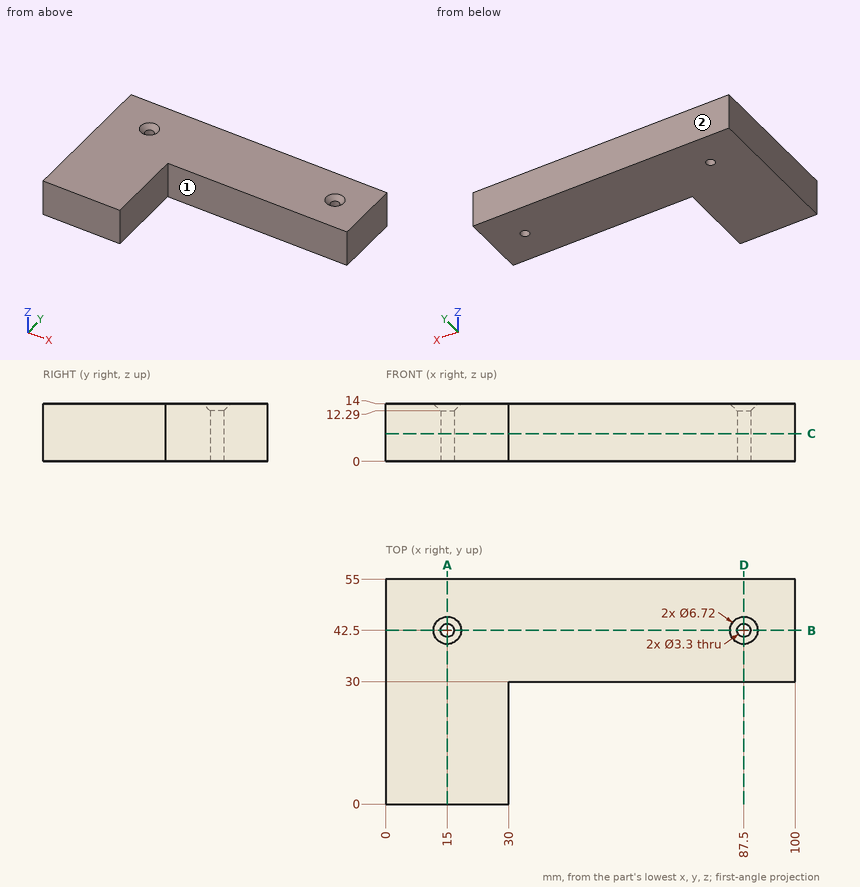
Could you check a few things on this drawing? It's one solid part, dimensions in mm from its lowest x, y, z. A direction names the side the tool comes from. Give positions to 0.01 mm unless a question says otherwise; leave off trailing zeros. Write each loop counter-clockwise with the first axis right and the second up, starting at its lowest first coordinate (ties: lowest second). Pieces come first, ordered by that corner, then holes. Notation, with made-up numbers: (35.5, 24.5) -> (87.5, 24.5) arc R16 cw to (87.5, 48.5) -> close; hole circle Ø5 at (-2.5, 63). An arc over 180 degrees is marked (long way). Answer as a JSON object with one key per item and string values.
Q1. Suppose I cut it at A-A on x = 15. Write out the boundary of the cut face in (y, z).
Taken from the geometry:
{"outline": "(0, 0) -> (40.85, 0) -> (40.85, 12.29) -> (39.14, 14) -> (0, 14) -> close; (44.15, 0) -> (55, 0) -> (55, 14) -> (45.86, 14) -> (44.15, 12.29) -> close"}
Q2. Suppose I cut it at B-B on y = 42.5. Write out the boundary of the cut face in (x, z).
Taken from the geometry:
{"outline": "(0, 0) -> (13.35, 0) -> (13.35, 12.29) -> (11.64, 14) -> (0, 14) -> close; (16.65, 0) -> (85.85, 0) -> (85.85, 12.29) -> (84.14, 14) -> (18.36, 14) -> (16.65, 12.29) -> close; (89.15, 0) -> (100, 0) -> (100, 14) -> (90.86, 14) -> (89.15, 12.29) -> close"}
Q3. Suppose I cut it at C-C on z = 6.75. Write out the boundary of the cut face in (x, y).
Taken from the geometry:
{"outline": "(0, 0) -> (30, 0) -> (30, 30) -> (100, 30) -> (100, 55) -> (0, 55) -> close; hole circle Ø3.3 at (15, 42.5); hole circle Ø3.3 at (87.5, 42.5)"}
Q4. Which directions (+Z, -Z, +X, -X, +Y, -Y) give clear straight access to the entire face, cutting with the end or side of a thin tool? Please do the marked faces 1 and 2.
Taken from the geometry:
{"face 1": "+Z, -Z, +X, -Y", "face 2": "+Z, -Z, +X, -X, +Y"}
Q5. Please list where these lines run through material, in increasing order: L1, parallel to X at y = 42.5, z = 2.5; L2, parallel to Y at x = 15, z = 4.25; L3, parallel to Y at x = 79, z = 6.25.
Taken from the geometry:
{"L1": "x = 0 to 13.35, 16.65 to 85.85, 89.15 to 100", "L2": "y = 0 to 40.85, 44.15 to 55", "L3": "y = 30 to 55"}
Q6. Suppose I cut it at D-D on x = 87.5. Write out the boundary of the cut face in (y, z), then the cut area to 3 significant figures.
Taken from the geometry:
{"outline": "(30, 0) -> (40.85, 0) -> (40.85, 12.29) -> (39.14, 14) -> (30, 14) -> close; (44.15, 0) -> (55, 0) -> (55, 14) -> (45.86, 14) -> (44.15, 12.29) -> close", "area": "301 mm²"}
Q7. Will these pins go through, and if not, where does the flat tip stop? pin 1 Ø3 at (x, y) = (87.5, 42.5) entering from -Z; pin 2 Ø5 at (x, z) = (40, 8) entering from -Y; pin 3 Ø4 at (x, y) = (15, 42.5) entering from +Z; pin 4 Ø8 at (y, z) = (17, 11) entering from +X.
Taken from the geometry:
{"pin 1": "passes through", "pin 2": "stops at y = 30", "pin 3": "stops at z = 12.64", "pin 4": "stops at x = 30"}
